Could you check a few things on this model? Use its own coordinates, in mm. Face numbers are marked on the shaded views. A direction names the side the tool comes from. Give positions to 0.01 mm unless a question says otherwise; leave off trailing zeros. Order: outer loops, then holes, each group sorted by start corner. A loop starts at its lowest first (then second) coordinate and runs counter-clockwise, first axis right, second up. Notation, with made-up numbers: (28.25, -4.75) -> (43.25, -4.75) arc R5 cw to (43.25, 4.25) -> close; hole circle Ø1 at (26.5, -21.75). An arc over 180 degrees is marked (long way). One line per item, written item: value.
```python
from build123d import *

# Parameters (mm, degrees)
SKETCH_1_R          = 18.5
EXTRUDE_1_DEPTH     = 100
EXTRUDE_2_DEPTH     = 20
SKETCH_3_R          = 4
EXTRUDE_3_DEPTH     = 17
SKETCH_4_R          = 1.5
CUT_EXTRUDE_1_DEPTH = 3


with BuildPart() as part:
    # Эскиз1 → Бобышка-Вытянуть1 (new body)
    with BuildSketch(Plane.XY):
        Circle(SKETCH_1_R)
    extrude(amount=EXTRUDE_1_DEPTH)

    # Эскиз2 → Бобышка-Вытянуть2 (add)
    with BuildSketch(Plane.XY.offset(100)):
        with BuildLine():
            Line((0, 18.5), (-22.5, 18.5))
            Line((-22.5, 18.5), (-22.5, -18.5))
            Line((-22.5, -18.5), (0, -18.5))
            ThreePointArc((0, -18.5), (18.5, 0), (0, 18.5))
        make_face()
    extrude(amount=EXTRUDE_2_DEPTH)

    # Эскиз3 → Бобышка-Вытянуть3 (add)
    with BuildSketch(Plane(origin=(0, 0, 0), x_dir=(-1, 0, 0), z_dir=(0, 0, -1))):
        Circle(SKETCH_3_R)
    extrude(amount=EXTRUDE_3_DEPTH)

    # Эскиз4 → Вырез-Вытянуть1 (cut)
    with BuildSketch(Plane(origin=(0, 0, 0), x_dir=(-1, 0, 0), z_dir=(0, 0, -1))):
        with Locations((15, 0)):
            Circle(SKETCH_4_R)
        with Locations((0, 15)):
            Circle(SKETCH_4_R)
        with Locations((-15, 0)):
            Circle(SKETCH_4_R)
        with Locations((0, -15)):
            Circle(SKETCH_4_R)
    extrude(amount=-CUT_EXTRUDE_1_DEPTH, mode=Mode.SUBTRACT)


solid = part.part
```
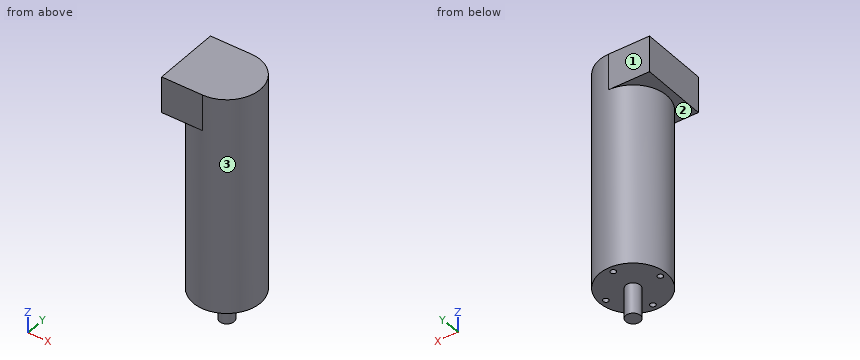
1) Suppose I cut it at C-C, the plane x = -10.5. Write out the boundary of the cut face in (y, z), then the cut area to 3 significant figures.
Answer below:
outline: (-18.5, 100) -> (-15.23, 100) -> (-15.23, 0) -> (15.23, 0) -> (15.23, 100) -> (18.5, 100) -> (18.5, 120) -> (-18.5, 120) -> close
area: 3,790 mm2
2) For the marked faces 1, 2 and 3, which set-ups out of +Z, -Z, +X, -X, +Y, -Y let a thin tool reach every point of the face, with its end or its side?
Answer below:
face 1: +Z, -Z, +X, -X, +Y
face 2: -Z, -X
face 3: -Z
3) Suppose I cut it at D-D, the plane y = -15. Write out the boundary of the cut face in (x, z), then the cut area to 3 significant figures.
Answer below:
outline: (-22.5, 100) -> (-10.83, 100) -> (-10.83, 0) -> (-1.5, 0) -> (-1.5, 3) -> (1.5, 3) -> (1.5, 0) -> (10.83, 0) -> (10.83, 120) -> (-22.5, 120) -> close
area: 2,820 mm2
4) Suppose I cut it at A-A, the plane y = 0. Write out the boundary of the cut face in (x, z).
Answer below:
outline: (-22.5, 100) -> (-18.5, 100) -> (-18.5, 0) -> (-16.5, 0) -> (-16.5, 3) -> (-13.5, 3) -> (-13.5, 0) -> (-4, 0) -> (-4, -17) -> (4, -17) -> (4, 0) -> (13.5, 0) -> (13.5, 3) -> (16.5, 3) -> (16.5, 0) -> (18.5, 0) -> (18.5, 120) -> (-22.5, 120) -> close
5) Suppose I cut it at B-B, the plane z = -4. Write out the boundary of the cut face in (x, y).
Answer below:
outline: circle Ø8 at (0, 0)
6) For P1, Ø1.5, axis at x = 15.5, y = 0, coming from the -Z side; P2, Ø2.5, axis at x = -0.5, y = 14.5, coming from the -Z side; P3, Ø2, axis at x = -13, z = 62.5, coming from the +Y side, each with a flat end and sliding along its axis, tell me the tip position at first contact or that it passes through.
Answer below:
P1: stops at z = 3
P2: stops at z = 0
P3: stops at y = 14.08
7) If I drill on line 1 along Y through (x, z) = (0, 1.3); line 2 along Z through (x, y) = (-4, -8); line 3 along Y through (x, z) = (1, 63), over which ranges is the centre line in solid material (lowest first)?
Answer below:
line 1: y = -18.5 to -16.5, -13.5 to 13.5, 16.5 to 18.5
line 2: z = 0 to 120
line 3: y = -18.47 to 18.47
